Can you work these out from the model? Positions are in its coordinate system, mm. A direction names the side the tool comes from. Round coordinates to 2 decimals unless told otherwise and drop trailing zeros. Order: outer loops, then holes, each group sorted by start corner. A loop starts at its lowest first (then second) coordinate and runs counter-clockwise, first axis right, second up. Notation, with made-up numbers: M -0.5,-22.75 L 33.5,-22.75 A34 cw 33.5,11.25 Z; hole C 31.25,49 d7. An arc over 180 degrees is marked long. Answer as a JSON object with one key per item and string values. Group by question number.
```python
from build123d import *

# Parameters (mm, degrees)
F0_R     = 3.25
F1_DEPTH = 3


with BuildPart() as f1:
    # F0 (on Front) → F1 (new body)
    with BuildSketch(Plane.XZ):
        Polygon((3, 2.8), (3, 0), (3, -2.8), (0, -2.8), (0, -12.8), (3, -12.8), (3, -19.8), (20, -19.8), (20, -22.8), (30, -22.8), (30, -19.8), (39, -19.8), (39, -13.3), (38, -13.3), (38, -11.3), (39, -11.3), (39, -7.8), (41, -7.8), (41, -11.3), (42, -11.3), (42, -13.3), (41, -13.3), (41, -19.8), (50, -19.8), (50, -22.8), (55, -22.8), (60, -22.8), (60, -19.8), (69, -19.8), (69, -13.3), (68, -13.3), (68, -11.3), (69, -11.3), (69, -7.8), (71, -7.8), (71, -11.3), (72, -11.3), (72, -13.3), (71, -13.3), (71, -19.8), (80, -19.8), (80, -22.8), (90, -22.8), (90, -19.8), (107, -19.8), (107, -12.8), (110, -12.8), (110, -2.8), (107, -2.8), (107, 0), (107, 2.8), (110, 2.8), (110, 12.8), (107, 12.8), (107, 19.8), (90, 19.8), (90, 22.8), (80, 22.8), (80, 19.8), (71, 19.8), (71, 13.3), (72, 13.3), (72, 11.3), (71, 11.3), (71, 7.8), (69, 7.8), (69, 11.3), (68, 11.3), (68, 13.3), (69, 13.3), (69, 19.8), (60, 19.8), (60, 22.8), (55, 22.8), (50, 22.8), (50, 19.8), (41, 19.8), (41, 13.3), (42, 13.3), (42, 11.3), (41, 11.3), (41, 7.8), (39, 7.8), (39, 11.3), (38, 11.3), (38, 13.3), (39, 13.3), (39, 19.8), (30, 19.8), (30, 22.8), (20, 22.8), (20, 19.8), (3, 19.8), (3, 12.8), (0, 12.8), (0, 2.8), align=None)
        with Locations((90.25, 0)):
            Circle(F0_R, mode=Mode.SUBTRACT)
    extrude(amount=F1_DEPTH)


solid = f1.part
```
1) If we section it at A-A on z = 0: Write out the boundary of the cut face in (x, y).
2) For pin 1 (0.9 mm diameter, centred on y = -1, z = -18, fed in from -X); pin 2 (1.5 mm diameter, centred on x = 108, y = -2, fed in from +Z); pin 3 (0.6 mm diameter, centred on x = 40.5, y = -1, fed in from +Z), each with a flat end and sliding along its axis, tell me the tip position at first contact or that it passes through.
3) If we section it at D-D on x = 78: Write out the boundary of the cut face in (y, z), plus the area to 3 significant figures.
4) If we section it at C-C on z = 14.5: Write out the boundary of the cut face in (x, y), plus the area to 3 significant figures.
5) We'd pull the mould along X, two halves only. Please class faces 4 (the face through (108, -1, 2.8)), 5 (the face through (41, -1, -17)), 6 (the face through (0, -1, 8)): +X half, -X half, draft (parallel to the pull), parting line (faces both ways), or undercut.
6) If we section it at B-B on z = -9: Write out the boundary of the cut face in (x, y).
7) I need wall thicknesses on line 1 along X through (y, z) = (-1.15, -20); line 2 along X through (y, z) = (-2.15, 11); line 3 along Z through (x, y) = (90.25, -1.3). Which ranges of each line are inside material? Lowest first, please.
8) Which directions (+Z, -Z, +X, -X, +Y, -Y) give clear straight access to the entire face, cutting with the end or side of a thin tool? Please do faces 1 (the face through (98, -1, -19.8)), 2 (the face through (38, -1, 12)), 3 (the face through (45, -1, -19.8)).
Findings:
{
 "1": {"outline": "M 3,-3 L 87,-3 L 87,0 L 3,0 Z; M 93.5,-3 L 107,-3 L 107,0 L 93.5,0 Z"},
 "2": {"pin 1": "stops at x = 3", "pin 2": "stops at z = 12.8", "pin 3": "stops at z = 7.8"},
 "3": {"outline": "M -3,-19.8 L 0,-19.8 L 0,19.8 L -3,19.8 Z", "area": "119 mm^2"},
 "4": {"outline": "M 3,-3 L 39,-3 L 39,0 L 3,0 Z; M 41,-3 L 69,-3 L 69,0 L 41,0 Z; M 71,-3 L 107,-3 L 107,0 L 71,0 Z", "area": "300 mm^2"},
 "5": {"face 4": "draft", "face 5": "undercut", "face 6": "-X half"},
 "6": {"outline": "M 0,-3 L 39,-3 L 39,0 L 0,0 Z; M 41,-3 L 69,-3 L 69,0 L 41,0 Z; M 71,-3 L 110,-3 L 110,0 L 71,0 Z"},
 "7": {"line 1": "x = 20 to 30, 50 to 60, 80 to 90", "line 2": "x = 0 to 39, 41 to 69, 71 to 110", "line 3": "z = -19.8 to -3.25, 3.25 to 19.8"},
 "8": {"face 1": "-Z, +X, +Y, -Y", "face 2": "+Y, -Y", "face 3": "-Z, +Y, -Y"}
}
